Verification items for this drawing (mm, ordinates from the low corner). Coordinates: 2 decimals unless noted, no trailing zeros. Loops run counter-clockwise (first coordinate to the right, second up) from the corner with the lowest first, then second, coordinate; pieces in that order, holes last. Notation, with made-up numbers: M 9,38 L 50,38 A23 cw 50,63 Z; hole C 21.25,55.5 d8. An arc over 180 degrees is marked long. Return JSON: item names as keys, results as strings.
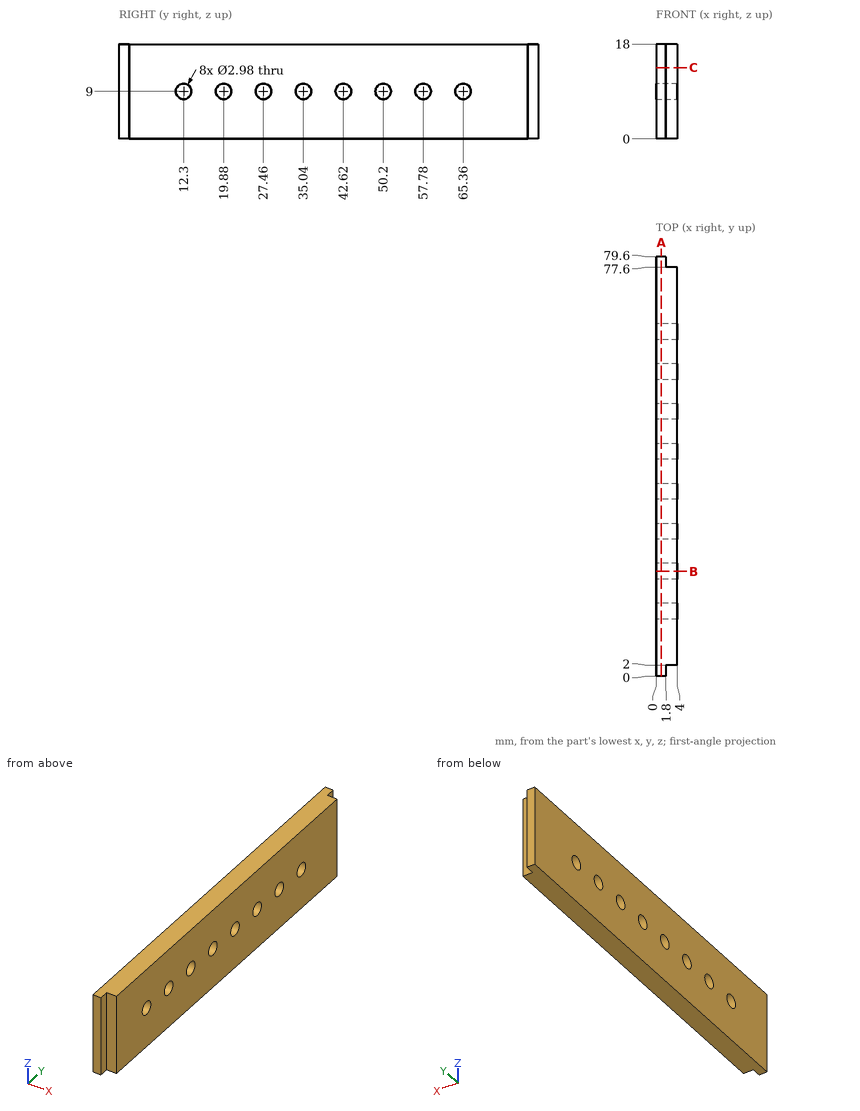
1) Section check A-A on x = 1. Count the separate pieces of the cut face and the enclosed holes in it, then the cut area to 3 significant figures.
Answers:
{"separate pieces": "1", "enclosed holes": "8", "area": "1,380 mm²"}
2) Go/stop test with flat-tipped pins: pin 1 Ø0.6 at (y, z) = (0.5, 10) entering from +X; pin 2 Ø1 at (x, z) = (2.5, 2.5) entering from -Y; pin 3 Ø1.1 at (x, z) = (2.5, 12.5) entering from +Y. Record where each tip stops, or that it passes through.
Answers:
{"pin 1": "x = 1.8", "pin 2": "y = 2", "pin 3": "y = 77.6"}
3) Section check B-B on y = 19.88. Record the cut outline in (x, z).
Answers:
{"outline": "M 0,0 L 4,0 L 4,7.51 L 0,7.51 Z; M 0,10.49 L 4,10.49 L 4,18 L 0,18 Z"}
4) Section check C-C on z = 13.5. Record the cut outline in (x, y).
Answers:
{"outline": "M 0,0 L 1.8,0 L 1.8,2 L 4,2 L 4,77.6 L 1.8,77.6 L 1.8,79.6 L 0,79.6 Z"}
5) Scan lines: line 1 along Z through (x, y) = (2.75, 57.78); line 2 along Y through (x, z) = (3.4, 11); line 3 along Z through (x, y) = (1.75, 34.5). Record each from-to range of solid material in increasing order. Write a range as [from, to].
Answers:
{"line 1": "[0, 7.51], [10.49, 18]", "line 2": "[2, 77.6]", "line 3": "[0, 7.61], [10.39, 18]"}
